The model under review builds one solid part; all positions refer to its coordinate system, in mm. A direction names the side the tool comes from. Round coordinates to 2 decimals unless told otherwise and drop trailing zeros. Loops run counter-clockwise (first coordinate to the right, second up) from the corner with the lowest first, then second, coordinate; pieces in that order, holes last. Notation, with made-up numbers: (37, 73.5) -> (94, 73.5) arc R18 cw to (94, 77.5) -> close; hole circle Ø11 at (82.25, -28). An arc over 180 degrees is marked (long way). Use a Markdown table: item, result. Add a question column.
1) Consider section B-B on x = -6. Give the boundary of the cut face in (y, z), plus the area to 3 significant figures.
2) Consider section D-D on y = 3.5. Give the boundary of the cut face in (x, z), plus the area to 3 significant figures.
3) For faces 5 (the cylindrical face through (19.09, -25.24, 2.25)), 6 (the flat face through (-27, -52.602, 1)), 7 (the flat face through (-30.84, -17.1, 2.6)), list the 3-axis set-ups (+Z, -Z, +X, -X, +Y, -Y) from which the entire face can be reached by the end or side of a thin tool; tool diameter is ignored.
4) Consider section A-A on y = -38. Give the boundary of the cut face in (x, z).
5) Insertion check: pin 1 (2.5 mm diameter, centred on x = 20.16, y = -49.8, fed in from +Z); pin 2 (1.1 mm diameter, centred on x = -4, y = 23, fed in from +Z); pin 3 (0.5 mm diameter, centred on x = 24, z = 0.5, fed in from -Y); pin 4 (0.7 mm diameter, centred on x = -27.5, z = 2.5, fed in from +Y). Each pin has a flat end and moves straight along its axis. Give the tip position at first contact, or say it passes through.
6) Consider section C-C on z = 1.1. State how many separate pieces and enclosed holes the cut face has, plus the area to 3 significant figures.
7) Wall thickness on probe 1 along Y at (x, z) = (-25.5, 1.55); probe 2 along Y at (x, z) = (14, 2.05); probe 3 along Y at (x, z) = (20, 2.95): over which ranges is each line inside the solid? List them lowest first.
8) Mouldability with a two-part tool opening along Y and no side actions: class faces 1 (the cylindrical face through (-30.41, -53.3, 2.17)), 2 (the cylindrical face through (23.734, 21.795, 2.169)), 3 (the flat face through (22.6, 16.92, 1.18)), 4 (the flat face through (-29, 13.298, 3)) as released by +Y, released by -Y, zero draft, split by the parting line, or undercut.
from build123d import *

# Parameters (mm, degrees)
F1_DEPTH = 2.4
F2_R     = 1.5
F3_DEPTH = 2
F4_DEPTH = 0.4
F2_W     = 37
F2_H     = 1
F5_DEPTH = 0.6
F7_DEPTH = 4.4
F9_DEPTH = 0.5


with BuildPart() as f1:
    # F0 (on Top) → F1 (new body)
    with BuildSketch(Plane.XY):
        with BuildLine():
            Line((20.160271, 23.298074), (-26.839729, 23.298074))
            ThreePointArc((-26.839729, 23.298074), (-30.375263, 21.833608), (-31.839729, 18.298074))
            Line((-31.839729, 18.298074), (-31.839729, -49.801926))
            ThreePointArc((-31.839729, -49.801926), (-30.375263, -53.33746), (-26.839729, -54.801926))
            Line((-26.839729, -54.801926), (20.160271, -54.801926))
            ThreePointArc((20.160271, -54.801926), (23.695805, -53.33746), (25.160271, -49.801926))
            Line((25.160271, -49.801926), (25.160271, 18.298074))
            ThreePointArc((25.160271, 18.298074), (23.695805, 21.833608), (20.160271, 23.298074))
        make_face()
        Polygon((-30.072891, -49.801926), (-28.45631, -47.001926), (-25.223148, -47.001926), (-23.606568, -49.801926), (-25.223148, -52.601926), (-28.45631, -52.601926), align=None, mode=Mode.SUBTRACT)
        Polygon((16.927109, -49.801926), (18.54369, -47.001926), (21.776852, -47.001926), (23.393432, -49.801926), (21.776852, -52.601926), (18.54369, -52.601926), align=None, mode=Mode.SUBTRACT)
        Polygon((-30.072891, 18.298074), (-28.45631, 21.098074), (-25.223148, 21.098074), (-23.606568, 18.298074), (-25.223148, 15.498074), (-28.45631, 15.498074), align=None, mode=Mode.SUBTRACT)
        Polygon((16.927109, 18.298074), (18.54369, 21.098074), (21.776852, 21.098074), (23.393432, 18.298074), (21.776852, 15.498074), (18.54369, 15.498074), align=None, mode=Mode.SUBTRACT)
    extrude(amount=F1_DEPTH)

    # F2 (on face) → F3 (join)
    with BuildSketch(Plane.XY.offset(2.4)):
        with BuildLine():
            Line((-21.839729, 23.298074), (-26.839729, 23.298074))
            ThreePointArc((-26.839729, 23.298074), (-30.375263, 21.833608), (-31.839729, 18.298074))
            Line((-31.839729, 18.298074), (-31.839729, 13.298074))
            Line((-31.839729, 13.298074), (-30.839729, 13.298074))
            Line((-30.839729, 13.298074), (-26.839729, 13.298074))
            ThreePointArc((-26.839729, 13.298074), (-23.304195, 14.76254), (-21.839729, 18.298074))
            Line((-21.839729, 18.298074), (-21.839729, 22.298074))
            Line((-21.839729, 22.298074), (-21.839729, 23.298074))
        make_face()
        Polygon((-28.45631, 15.498074), (-30.072891, 18.298074), (-28.45631, 21.098074), (-25.223148, 21.098074), (-23.606568, 18.298074), (-25.223148, 15.498074), align=None, mode=Mode.SUBTRACT)
        with BuildLine():
            Line((20.160271, 23.298074), (15.160271, 23.298074))
            Line((15.160271, 23.298074), (15.160271, 22.298074))
            Line((15.160271, 22.298074), (15.160271, 18.298074))
            ThreePointArc((15.160271, 18.298074), (16.624737, 14.76254), (20.160271, 13.298074))
            Line((20.160271, 13.298074), (24.160271, 13.298074))
            Line((24.160271, 13.298074), (25.160271, 13.298074))
            Line((25.160271, 13.298074), (25.160271, 18.298074))
            ThreePointArc((25.160271, 18.298074), (23.695805, 21.833608), (20.160271, 23.298074))
        make_face()
        Polygon((23.393432, 18.298074), (21.776852, 15.498074), (18.54369, 15.498074), (16.927109, 18.298074), (18.54369, 21.098074), (21.776852, 21.098074), align=None, mode=Mode.SUBTRACT)
        with BuildLine():
            Line((25.160271, -49.801926), (25.160271, -44.801926))
            Line((25.160271, -44.801926), (24.160271, -44.801926))
            Line((24.160271, -44.801926), (24.160271, -46.590926))
            Line((24.160271, -46.590926), (16.327585, -46.590926))
            ThreePointArc((16.327585, -46.590926), (15.461152, -48.093627), (15.160271, -49.801926))
            Line((15.160271, -49.801926), (15.160271, -53.801926))
            Line((15.160271, -53.801926), (15.160271, -54.801926))
            Line((15.160271, -54.801926), (20.160271, -54.801926))
            ThreePointArc((20.160271, -54.801926), (23.695805, -53.33746), (25.160271, -49.801926))
        make_face()
        Polygon((18.54369, -52.601926), (16.927109, -49.801926), (18.54369, -47.001926), (21.776852, -47.001926), (23.393432, -49.801926), (21.776852, -52.601926), align=None, mode=Mode.SUBTRACT)
        with BuildLine():
            Line((-30.839729, -44.801926), (-31.839729, -44.801926))
            Line((-31.839729, -44.801926), (-31.839729, -49.801926))
            ThreePointArc((-31.839729, -49.801926), (-30.375263, -53.33746), (-26.839729, -54.801926))
            Line((-26.839729, -54.801926), (-21.839729, -54.801926))
            Line((-21.839729, -54.801926), (-21.839729, -53.801926))
            Line((-21.839729, -53.801926), (-21.839729, -49.801926))
            ThreePointArc((-21.839729, -49.801926), (-22.140611, -48.093627), (-23.007044, -46.590926))
            Line((-23.007044, -46.590926), (-30.839729, -46.590926))
            Line((-30.839729, -46.590926), (-30.839729, -44.801926))
        make_face()
        Polygon((-25.223148, -52.601926), (-28.45631, -52.601926), (-30.072891, -49.801926), (-28.45631, -47.001926), (-25.223148, -47.001926), (-23.606568, -49.801926), align=None, mode=Mode.SUBTRACT)
        Polygon((-30.072891, -49.801926), (-28.45631, -52.601926), (-25.223148, -52.601926), (-23.606568, -49.801926), (-25.223148, -47.001926), (-28.45631, -47.001926), align=None)
        with Locations((-26.839729, -49.801926)):
            Circle(F2_R, mode=Mode.SUBTRACT)
        Polygon((18.54369, -47.001926), (16.927109, -49.801926), (18.54369, -52.601926), (21.776852, -52.601926), (23.393432, -49.801926), (21.776852, -47.001926), align=None)
        with Locations((20.160271, -49.801926)):
            Circle(F2_R, mode=Mode.SUBTRACT)
        Polygon((18.54369, 15.498074), (21.776852, 15.498074), (23.393432, 18.298074), (21.776852, 21.098074), (18.54369, 21.098074), (16.927109, 18.298074), align=None)
        with Locations((20.160271, 18.298074)):
            Circle(F2_R, mode=Mode.SUBTRACT)
        Polygon((-28.45631, 21.098074), (-30.072891, 18.298074), (-28.45631, 15.498074), (-25.223148, 15.498074), (-23.606568, 18.298074), (-25.223148, 21.098074), align=None)
        with Locations((-26.839729, 18.298074)):
            Circle(F2_R, mode=Mode.SUBTRACT)
    extrude(amount=F3_DEPTH)

    # F2 (on face) → F4 (cut)
    with BuildSketch(Plane.XY.offset(2.4)):
        with BuildLine():
            Line((15.160271, 22.298074), (-21.839729, 22.298074))
            Line((-21.839729, 22.298074), (-21.839729, 18.298074))
            ThreePointArc((-21.839729, 18.298074), (-23.304195, 14.76254), (-26.839729, 13.298074))
            Line((-26.839729, 13.298074), (-30.839729, 13.298074))
            Line((-30.839729, 13.298074), (-30.839729, -43.238085))
            Line((-30.839729, -43.238085), (-30.839729, -44.801926))
            Line((-30.839729, -44.801926), (-30.839729, -46.590926))
            Line((-30.839729, -46.590926), (-23.007044, -46.590926))
            ThreePointArc((-23.007044, -46.590926), (-22.140611, -48.093627), (-21.839729, -49.801926))
            Line((-21.839729, -49.801926), (-21.839729, -53.801926))
            Line((-21.839729, -53.801926), (15.160271, -53.801926))
            Line((15.160271, -53.801926), (15.160271, -49.801926))
            ThreePointArc((15.160271, -49.801926), (15.461152, -48.093627), (16.327585, -46.590926))
            Line((16.327585, -46.590926), (24.160271, -46.590926))
            Line((24.160271, -46.590926), (24.160271, -44.801926))
            Line((24.160271, -44.801926), (24.160271, -43.238085))
            Line((24.160271, -43.238085), (24.160271, 13.298074))
            Line((24.160271, 13.298074), (20.160271, 13.298074))
            ThreePointArc((20.160271, 13.298074), (16.624737, 14.76254), (15.160271, 18.298074))
            Line((15.160271, 18.298074), (15.160271, 22.298074))
        make_face()
    extrude(amount=-F4_DEPTH, mode=Mode.SUBTRACT)

    # F2 (on face) → F5 (join)
    with BuildSketch(Plane.XY.offset(2.4)):
        Polygon((-30.839729, 13.298074), (-31.839729, 13.298074), (-31.839729, -44.801926), (-30.839729, -44.801926), (-30.839729, -43.238085), align=None)
        with Locations((-3.339729, 22.798074)):
            Rectangle(F2_W, F2_H)
        Polygon((25.160271, -44.801926), (25.160271, 13.298074), (24.160271, 13.298074), (24.160271, -43.238085), (24.160271, -44.801926), align=None)
        with Locations((-3.339729, -54.301926)):
            Rectangle(F2_W, F2_H)
    extrude(amount=F5_DEPTH)

    # F6 (on face) → F7 (cut)
    with BuildSketch(Plane(origin=(0, 0, 0), x_dir=(1, 0, 0), z_dir=(0, 0, -1))):
        Polygon((24.160271, 19.590926), (25.160271, 19.590926), (25.160271, 46.590926), (24.160271, 46.590926), (24.160271, 48.590926), (23.160271, 48.590926), (23.160271, 46.590926), (23.160271, 19.590926), (23.160271, 17.590926), (24.160271, 17.590926), align=None)
    extrude(amount=-F7_DEPTH, mode=Mode.SUBTRACT)

    # F8 (on face) → F9 (join)
    with BuildSketch(Plane.XY.offset(2)):
        with BuildLine():
            ThreePointArc((19.663978, -26.639785), (19.078192, -25.225571), (17.663978, -24.639785))
            Line((17.663978, -24.639785), (-24.344087, -24.639785))
            ThreePointArc((-24.344087, -24.639785), (-25.758301, -25.225571), (-26.344087, -26.639785))
            Line((-26.344087, -26.639785), (-26.344087, -39.868281))
            ThreePointArc((-26.344087, -39.868281), (-25.758301, -41.282494), (-24.344087, -41.868281))
            Line((-24.344087, -41.868281), (17.663978, -41.868281))
            ThreePointArc((17.663978, -41.868281), (19.078192, -41.282494), (19.663978, -39.868281))
            Line((19.663978, -39.868281), (19.663978, -26.639785))
        make_face()
    extrude(amount=F9_DEPTH)


solid = f1.part
Result set:
| question | item | result |
|---|---|---|
| 1 | outline | (-54.8, 0) -> (23.3, 0) -> (23.3, 3) -> (22.3, 3) -> (22.3, 2) -> (-24.64, 2) -> (-24.64, 2.5) -> (-41.87, 2.5) -> (-41.87, 2) -> (-53.8, 2) -> (-53.8, 3) -> (-54.8, 3) -> close |
| 1 | area | 167 mm2 |
| 2 | outline | (-31.84, 0) -> (25.16, 0) -> (25.16, 3) -> (24.16, 3) -> (24.16, 2) -> (-30.84, 2) -> (-30.84, 3) -> (-31.84, 3) -> close |
| 2 | area | 116 mm2 |
| 3 | face 5 | +Z, +X |
| 3 | face 6 | -Z |
| 3 | face 7 | +Z |
| 4 | outline | (-31.84, 0) -> (23.16, 0) -> (23.16, 2) -> (19.66, 2) -> (19.66, 2.5) -> (-26.34, 2.5) -> (-26.34, 2) -> (-30.84, 2) -> (-30.84, 3) -> (-31.84, 3) -> close |
| 5 | pin 1 | through |
| 5 | pin 2 | z = 3 |
| 5 | pin 3 | y = -53.28 |
| 5 | pin 4 | y = 23.29 |
| 6 | separate pieces | 1 |
| 6 | enclosed holes | 4 |
| 6 | area | 4,260 mm2 |
| 7 | probe 1 | -54.8 to -52.6, -47 to 15.5, 21.1 to 23.3 |
| 7 | probe 2 | -54.8 to -53.8, -41.87 to -24.64, 22.3 to 23.3 |
| 7 | probe 3 | -54.8 to -51.29, -48.31 to -46.59, 13.3 to 16.81, 19.79 to 23.3 |
| 8 | face 1 | released by -Y |
| 8 | face 2 | released by +Y |
| 8 | face 3 | undercut |
| 8 | face 4 | undercut |
